Geometry: final body of the model. Coordinates: model frame, mm. Give positions to 0.01 mm unless a question says otherwise; leave off trailing zeros. Loops run counter-clockwise (first coordinate to the right, second up) from the corner with the lowest first, then second, coordinate; pieces in that order, holes last.
1. Material intervals for line 1 along X through (y, z) = (5, 1); line 2 along X through (y, z) = (-4, 0.95); line 3 along Y through (x, z) = (-19, 0.8), sorted ascending.
2. Section D-D, the plane y = -4. Output: boundary loops of the cut face in (x, z), then the cut area to 3 significant figures.
3. Section A-A, the plane y = 5. Output: boundary loops of the cut face in (x, z), then the cut area to 3 significant figures.
4. First-contact query: P1, Ø1.3, axis at x = 24, y = -4, coming from the +Z side; P2, Ø0.5, axis at x = -7, z = 1, coming from the +Y side. Flat tips, straight axial feed; report the tip coordinate or a pass-through.
5. Section B-B, the plane x = 36. Output: boundary loops of the cut face in (y, z), then the cut area to 3 significant figures.
6. Section C-C, the plane z = 1.25. Output: boundary loops of the cut face in (x, y).
Autodesk Inventor part; units mm, degrees
ref_plane "YZ Plane" through (0, 0, 0) normal (1, 0, 0) x (0, 1, 0)
ref_plane "XZ Plane" through (0, 0, 0) normal (0, 1, 0) x (-1, 0, 0)
ref_plane "XY Plane" through (0, 0, 0) normal (0, 0, 1) x (1, 0, 0)
sketch "Skizze1" plane through (0, 0, 0) normal (0, 0, 1) x (1, 0, 0)
  line L0 (-41, -7) -> (41, -7)
  line L1 (41, -7) -> (41, 7)
  line L2 (-41, 7) -> (-41, -7)
  line L3 (-41, -7) -> (41, 7) construction
  line L4 (41, -7) -> (-41, 7) construction
  line L5 (16.3, 7) -> (16.3, 2.8)
  line L6 (16.3, 2.8) -> (-16.3, 2.8)
  line L7 (-16.3, 2.8) -> (-16.3, 7)
  line L8 (41, 7) -> (16.3, 7)
  line L9 (-16.3, 7) -> (-41, 7)
  line L10 (0, 9.8) -> (0, -9.8)
  point P0 (0, 0)
  dimension "d0" = 82
  dimension "d1" = 14
  dimension "d13" = 4.2
  dimension "d14" = 32.6
extrude "Extrusion1" add sketch "Skizze1" along normal blind 1.6
sketch "Skizze2" plane through (0, 0, 1.6) normal (0, 0, 1) x (1, 0, 0)
  line L0 (0, 9.8) -> (0, -9.8)
  line L1 (-57.4, 0) -> (57.4, 0)
  line L2 (-19, 5) -> (19, 5) construction
  line L3 (-16.3, 7) -> (-41, 7)
  point P0 (0, 0)
  dimension "d4" = 38
  dimension "d15" = 2
hole "Bohrung1" at (-19, 5, 1.6) at (19, 5, 1.6) direction (0, 0, -1) diameter 2.1 end through all
sketch "Skizze3" plane through (0, 0, 1.6) normal (0, 0, 1) x (1, 0, 0)
  line L0 (-41, -7) -> (41, -7)
  line L1 (0, 9.8) -> (0, -9.8)
  line L2 (-36, -4) -> (-24, -4) construction
  line L3 (24, -4) -> (36, -4) construction
  point P0 (0, 0)
  dimension "d16" = 3
  dimension "d17" = 24
  dimension "d18" = 12
hole "Bohrung2" at (-36, -4, 1.6) at (-24, -4, 1.6) at (24, -4, 1.6) at (36, -4, 1.6) direction (0, 0, -1) diameter 2.1 end through all
properties part number "Eyeboard" material "Phenolharz"
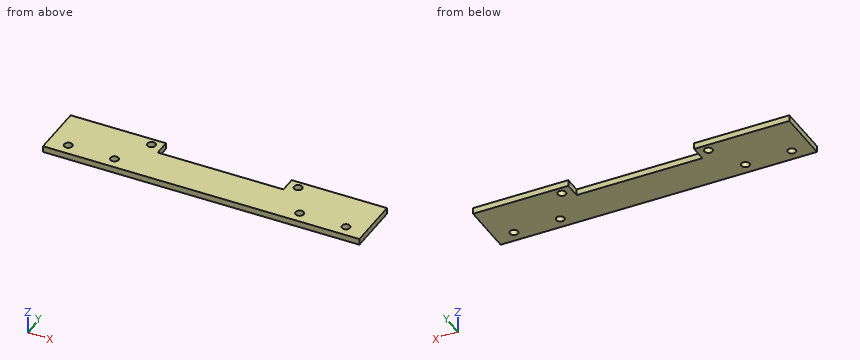
Answers below:
1. line 1: x = -41 to -20.05, -17.95 to -16.3, 16.3 to 17.95, 20.05 to 41
1. line 2: x = -41 to -37.05, -34.95 to -25.05, -22.95 to 22.95, 25.05 to 34.95, 37.05 to 41
1. line 3: y = -7 to 3.95, 6.05 to 7
2. outline: (-41, 0) - (-37.05, 0) - (-37.05, 1.6) - (-41, 1.6) - close; (-34.95, 0) - (-25.05, 0) - (-25.05, 1.6) - (-34.95, 1.6) - close; (-22.95, 0) - (22.95, 0) - (22.95, 1.6) - (-22.95, 1.6) - close; (25.05, 0) - (34.95, 0) - (34.95, 1.6) - (25.05, 1.6) - close; (37.05, 0) - (41, 0) - (41, 1.6) - (37.05, 1.6) - close
2. area: 118 mm2
3. outline: (-41, 0) - (-20.05, 0) - (-20.05, 1.6) - (-41, 1.6) - close; (-17.95, 0) - (-16.3, 0) - (-16.3, 1.6) - (-17.95, 1.6) - close; (16.3, 0) - (17.95, 0) - (17.95, 1.6) - (16.3, 1.6) - close; (20.05, 0) - (41, 0) - (41, 1.6) - (20.05, 1.6) - close
3. area: 72.3 mm2
4. P1: passes through
4. P2: stops at y = 2.8
5. outline: (-7, 0) - (-5.05, 0) - (-5.05, 1.6) - (-7, 1.6) - close; (-2.95, 0) - (7, 0) - (7, 1.6) - (-2.95, 1.6) - close
5. area: 19.0 mm2
6. outline: (-41, -7) - (41, -7) - (41, 7) - (16.3, 7) - (16.3, 2.8) - (-16.3, 2.8) - (-16.3, 7) - (-41, 7) - close; hole circle Ø2.1 at (-36, -4); hole circle Ø2.1 at (-24, -4); hole circle Ø2.1 at (-19, 5); hole circle Ø2.1 at (19, 5); hole circle Ø2.1 at (24, -4); hole circle Ø2.1 at (36, -4)
